Geometry check sheet. Reference: the model listing, model coordinates, mm. A direction names the side the tool comes from. Coordinates: 2 decimals unless noted, no trailing zeros. Order: outer loops, then holes, each group sorted by start corner. A loop starts at its lowest first (then second) coordinate and runs counter-clockwise, first axis right, second up. Notation, with made-up numbers: (4, -7.5) - (45, -7.5) arc R15 ccw to (45, 19.5) - close; hole circle Ø6 at (-5, 32.25). An arc over 180 degrees is marked (long way). Return JSON: item names as keys, results as strings. Group by question number.
Item 1: Gauge pin test, flat ends, axial feed: pin 1 (0.6 mm diameter, centred on y = -16, z = 20.5, fed in from +X); pin 2 (7 mm diameter, centred on x = -72, y = -6, fed in from +Z); pin 3 (1 mm diameter, centred on y = 9, z = 25, fed in from -X). Record the tip position at first contact, or that the pin passes through.
Item 2: Scan lines: probe 1 along Y at (x, z) = (-72, 21.6); probe 2 along Z at (x, y) = (-68.5, -9.5); probe 3 along X at (y, z) = (16.5, 22.75). Record each from-to range of solid material in increasing order.
Item 3: Section check A-A on y = -16. Enter the section's corners in (x, z), then the cut area to 3 significant figures.
Item 4: Section check D-D on x = -58. Enter the section's corners in (y, z).
Item 5: Section check C-C on y = -6. Enter the section's corners in (x, z), then the cut area to 3 significant figures.
Item 6: Tool access check on faces 1 (the flat face through (-69, 27.714, 28)), 2 (the flat face through (-60, -22.011, 21)), 3 (the flat face through (-61, 0, 21)). Record the directions out of +Z, -Z, +X, -X, +Y, -Y that give a thin tool (end or side, any length) a straight path to the whole face; none if there is none.
Item 7: Draft check along X on faces 4 (the flat face through (-54, -11, 21)), 5 (the flat face through (-60, -7.011, 21)), 6 (the flat face through (-75.5, -16, 21)). Enter one of: pulls with the +X half, pulls with the -X half, needs draft (parallel to the pull), parting line crosses it, or undercut.
Item 8: Section check B-B on x = -72. Enter the section's corners in (y, z), then the cut area to 3 significant figures.
from build123d import *

# Parameters (mm, degrees)
SKETCH028_R        = 2.25
SKETCH028_W        = 5
SKETCH028_H        = 15
PAD012_DEPTH       = 2
SKETCH029_W        = 2.5
SKETCH029_H        = 29.464039
PAD013_DEPTH       = 16
SKETCH030_R        = 2.5
POCKET007005_DEPTH = 18.151
POCKET007010_DEPTH = 5


with BuildPart() as part:
    # Sketch028 → Pad012 (new body)
    with BuildSketch(Plane.XY):
        Polygon((-52, -32), (-75.5, -32), (-75.5, 0), (-54, 0), (-54, -23.010657), (-52, -23.010657), align=None)
        with Locations((-72, -28)):
            Circle(SKETCH028_R, mode=Mode.SUBTRACT)
        with Locations((-72, -16)):
            Circle(SKETCH028_R, mode=Mode.SUBTRACT)
        with Locations((-72, -6)):
            Circle(SKETCH028_R, mode=Mode.SUBTRACT)
        with Locations((-57, -28)):
            Circle(SKETCH028_R, mode=Mode.SUBTRACT)
        with Locations((-59.5, -14.510657)):
            Rectangle(SKETCH028_W, SKETCH028_H, mode=Mode.SUBTRACT)
    extrude(amount=PAD012_DEPTH)

    # Sketch029 → Pad013 (join)
    with BuildSketch(Plane.XY):
        with Locations((-68.9, 12.982019)):
            Rectangle(SKETCH029_W, SKETCH029_H)
    extrude(amount=PAD013_DEPTH)

    # Sketch030 (on DatumPlane) → Pocket007005 (cut, through all)
    with BuildSketch(Plane(origin=(-70.15, -1.75, 0), x_dir=(0, 1, 0), z_dir=(1, 0, 0))):
        with Locations((24.414811, 10.983683)):
            Circle(SKETCH030_R)
    extrude(amount=POCKET007005_DEPTH, mode=Mode.SUBTRACT)

    # Sketch041 (on DatumPlane) → Pocket007010 (cut)
    with BuildSketch(Plane(origin=(-70.15, -1.75, 0), x_dir=(0, 1, 0), z_dir=(1, 0, 0))):
        Polygon((-2.326099, 2.494806), (28.94412, 20.456944), (-2.326099, 20.456944), align=None)
    extrude(amount=POCKET007010_DEPTH, mode=Mode.SUBTRACT)


with BuildPart() as part_1:
    # Body001 placement: moved
    add(part.part.moved(Location((0, 0, 20))))


solid = part_1.part
Computed:
{
 "1": {"pin 1": "stops at x = -54", "pin 2": "stops at z = 22", "pin 3": "stops at x = -70.15"},
 "2": {"probe 1": "y = -32 to -30.25, -25.75 to -18.25, -13.75 to -8.25, -3.75 to 0", "probe 2": "z = 20 to 22", "probe 3": "x = -70.15 to -67.65"},
 "3": {"outline": "(-75.5, 20) - (-74.25, 20) - (-74.25, 22) - (-75.5, 22) - close; (-69.75, 20) - (-62, 20) - (-62, 22) - (-69.75, 22) - close; (-57, 20) - (-54, 20) - (-54, 22) - (-57, 22) - close", "area": "24.0 mm²"},
 "4": {"outline": "(-32, 20) - (-30.02, 20) - (-30.02, 22) - (-32, 22) - close; (-25.98, 20) - (-22.01, 20) - (-22.01, 22) - (-25.98, 22) - close; (-7.01, 20) - (0, 20) - (0, 22) - (-7.01, 22) - close"},
 "5": {"outline": "(-75.5, 20) - (-74.25, 20) - (-74.25, 22) - (-75.5, 22) - close; (-69.75, 20) - (-54, 20) - (-54, 22) - (-69.75, 22) - close", "area": "34.0 mm²"},
 "6": {"face 1": "+Z, -Z, +X, -X, +Y", "face 2": "+Z, -Z", "face 3": "+Z, -Z, +X, +Y"},
 "7": {"face 4": "pulls with the +X half", "face 5": "undercut", "face 6": "pulls with the -X half"},
 "8": {"outline": "(-32, 20) - (-30.25, 20) - (-30.25, 22) - (-32, 22) - close; (-25.75, 20) - (-18.25, 20) - (-18.25, 22) - (-25.75, 22) - close; (-13.75, 20) - (-8.25, 20) - (-8.25, 22) - (-13.75, 22) - close; (-3.75, 20) - (0, 20) - (0, 22) - (-3.75, 22) - close", "area": "37.0 mm²"}
}
